```python
from build123d import *

# Parameters (mm, degrees)
CHAMFER1_SIZE      = 0.2
CUT_EXTRUDE1_DEPTH = 0.75


with BuildPart() as part:
    # Sketch1 → Revolve1 (revolve)
    with BuildSketch(Plane.XY):
        Polygon((0, 1), (-1, 2), (-1.2, 2), (-1.2, 0), (6.8, 0), (6.8, 1), align=None)
    revolve(axis=Axis((-1.2, 0, 0), (1, 0, 0)))

    # Chamfer1
    chamfer1_edges = [part.edges().sort_by_distance(p)[0] for p in [
        (6.8, -1, 0),
    ]]
    chamfer(chamfer1_edges, length=CHAMFER1_SIZE)

    # Sketch2 → Cut-Extrude1 (cut)
    with BuildSketch(Plane.ZY.offset(1.2)):
        Polygon((-0.75055535, 0), (-0.375277675, -0.65), (0.375277675, -0.65), (0.75055535, 0), (0.375277675, 0.65), (-0.375277675, 0.65), align=None)
    extrude(amount=-CUT_EXTRUDE1_DEPTH, mode=Mode.SUBTRACT)


solid = part.part
```
Read the model definition and answer for the solid it produces. Units are mm, in the model's axes. Give positions to 0.01 mm unless a question says otherwise; leave off trailing zeros. Order: outer loops, then holes, each group sorted by start corner. A loop starts at its lowest first (then second) coordinate and runs counter-clockwise, first axis right, second up.
(1) Find section B-B (x = 1). Give the vertices of the cut face in (y, z).
(2) Straight lines are drawn through the part: L1, parallel to Y at x = 0.5, z = -0.6; L2, parallel to X at y = 0.1, z = -0.2; L3, parallel to Y at x = 4.5, z = 0.05. For each, find the intervals that lie inside material, in ascending order.
(3) Given pin 1 (1 mm diameter, centred on y = -1, z = 1.5, fed in from +X); pin 2 (0.8 mm diameter, centred on x = -0.5, z = 0, fed in from -Y); pin 3 (0.7 mm diameter, centred on y = 0, z = 0, fed in from -X), each flat-ended and moving along its own axis, determine where each tip first touches the part or whether it passes through.
(4) Find section A-A (z = 0). Give the vertices of the cut face in (x, y), plus the area to 3 significant figures.
(5) For a pull along Y with two mould halves and no side action, classify faces 1 (the cylindrical face through (3, 0, -1)), 2 (the flat face through (-0.45, 0, 0)), 3 (the flat face through (6.8, 0, 0)) as released by +Y, released by -Y, zero draft, split by the parting line, or undercut.
Result sheet:
1. outline: circle Ø2 at (0, 0)
2. L1: y = -0.8 to 0.8
2. L2: x = -0.45 to 6.8
2. L3: y = -1 to 1
3. pin 1: stops at x = -0.3
3. pin 2: stops at y = -1.9
3. pin 3: stops at x = -0.45
4. outline: (-1.2, -2) - (-1, -2) - (0, -1) - (6.6, -1) - (6.8, -0.8) - (6.8, 0.8) - (6.6, 1) - (0, 1) - (-1, 2) - (-1.2, 2) - (-1.2, 0.65) - (-0.45, 0.65) - (-0.45, -0.65) - (-1.2, -0.65) - close
4. area: 16.4 mm2
5. face 1: split by the parting line
5. face 2: undercut
5. face 3: zero draft
